For this review, take the finished solid that the model builds, in its own axes (mm). Round coordinates to 2 decimals unless told otherwise and drop trailing zeros. Write each loop counter-clockwise with the first axis right and the second up, starting at its lowest first coordinate (ties: lowest second). Pieces come first, ordered by that corner, then holes. Notation, with made-up numbers: (-29.75, 52) - (-20.75, 52) arc R30 ccw to (-20.75, 84) - close; hole circle Ø5 at (11.5, -38). An arc over 180 degrees is marked (long way). One line per item, written item: value. Start each with the question number.
Q1. Add section A-A on x = 63.5. Write out the cut boundary in (y, z) (3 decimals).
Q2. Add section B-B on y = 12.7. Write out the cut boundary in (x, z) (3 decimals).
Q3. Add section D-D on y = 38.1. Write out the cut boundary in (x, z) (3 decimals).
Q4. For probe 1 along Y at (x, z) = (12.5, 0.15); probe 2 along Y at (x, z) = (36, 1.2); probe 3 along X at (y, z) = (48.5, 2.3), list the stretches that pass through material, from the lowest coordinate up.
Q5. Clearance check with flat-ended pins moving along their axes: pin 1 Ø10 at (x, y) = (44, 38.5) entering from -Z; pin 2 Ø1.6 at (x, z) = (9, 2.5) entering from +Y; pin 3 Ø1 at (y, z) = (38, 2) entering from +X; pin 4 Ø1.6 at (y, z) = (41, 1.5) entering from -X. State where each tip first meets the part, or that it passes through.
Q6. Add section C-C on z = 1.2. Write out the cut boundary in (x, y), and give its area (3 significant figures).
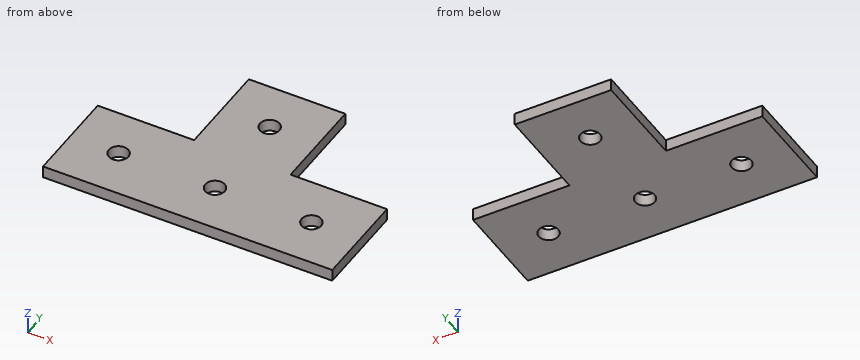
Autodesk Inventor part; units mm, degrees
ref_plane "YZ Plane" through (0, 0, 0) normal (1, 0, 0) x (0, 1, 0)
ref_plane "XZ Plane" through (0, 0, 0) normal (0, 1, 0) x (-1, 0, 0)
ref_plane "XY Plane" through (0, 0, 0) normal (0, 0, 1) x (1, 0, 0)
sketch "Sketch1" plane through (0, 0, 0) normal (0, 0, 1) x (1, 0, 0)
  line L0 (0, 0) -> (0, 25.4)
  line L1 (0, 25.4) -> (25.4, 25.4)
  line L2 (25.4, 25.4) -> (25.4, 50.8)
  line L3 (25.4, 50.8) -> (50.8, 50.8)
  line L4 (50.8, 50.8) -> (50.8, 25.4)
  line L5 (50.8, 25.4) -> (76.2, 25.4)
  line L6 (76.2, 25.4) -> (76.2, 0)
  line L7 (76.2, 0) -> (0, 0)
  line L8 (0, 12.7) -> (12.7, 12.7) construction
  line L9 (12.7, 12.7) -> (38.1, 12.7) construction
  line L10 (38.1, 12.7) -> (63.5, 12.7) construction
  line L11 (38.1, 12.7) -> (38.1, 38.1) construction
  circle A0 centre (38.1, 12.7) radius 2.5797
  circle A1 centre (63.5, 12.7) radius 2.5797
  circle A2 centre (12.7, 12.7) radius 2.5797
  circle A3 centre (38.1, 38.1) radius 2.5797
  dimension "d0" = 25.4
  dimension "d1" = 25.4
  dimension "d2" = 25.4
  dimension "d3" = 25.4
  dimension "d4" = 25.4
  dimension "d5" = 25.4
  dimension "d6" = 12.7
  dimension "d7" = 25.4
  dimension "d8" = 25.4
  dimension "d9" = 5.1594
extrude "Extrusion1" add sketch "Sketch1" along normal blind 3.175
properties part number "Short T-Gusset"
Result set:
1. outline: (0, 0) - (10.12, 0) - (10.12, 3.175) - (0, 3.175) - close; (15.28, 0) - (25.4, 0) - (25.4, 3.175) - (15.28, 3.175) - close
2. outline: (0, 0) - (10.12, 0) - (10.12, 3.175) - (0, 3.175) - close; (15.28, 0) - (35.52, 0) - (35.52, 3.175) - (15.28, 3.175) - close; (40.68, 0) - (60.92, 0) - (60.92, 3.175) - (40.68, 3.175) - close; (66.08, 0) - (76.2, 0) - (76.2, 3.175) - (66.08, 3.175) - close
3. outline: (25.4, 0) - (35.52, 0) - (35.52, 3.175) - (25.4, 3.175) - close; (40.68, 0) - (50.8, 0) - (50.8, 3.175) - (40.68, 3.175) - close
4. probe 1: y = 0 to 10.13, 15.27 to 25.4
4. probe 2: y = 0 to 11.2, 14.2 to 36.6, 39.6 to 50.8
4. probe 3: x = 25.4 to 50.8
5. pin 1: stops at z = 0
5. pin 2: stops at y = 25.4
5. pin 3: stops at x = 50.8
5. pin 4: stops at x = 25.4
6. outline: (0, 0) - (76.2, 0) - (76.2, 25.4) - (50.8, 25.4) - (50.8, 50.8) - (25.4, 50.8) - (25.4, 25.4) - (0, 25.4) - close; hole circle Ø5.16 at (12.7, 12.7); hole circle Ø5.16 at (38.1, 12.7); hole circle Ø5.16 at (38.1, 38.1); hole circle Ø5.16 at (63.5, 12.7)
6. area: 2,500 mm^2
